```python
from build123d import *

# Parameters (mm, degrees)
SKETCH1_W           = 20.3
SKETCH1_H           = 20.3
BOSS_EXTRUDE1_DEPTH = 39.3
FILLET1_R           = 1
SKETCH2_R           = 1
CUT_EXTRUDE1_DEPTH  = 2.5
SKETCH3_R           = 8
BOSS_EXTRUDE2_DEPTH = 1.5
SKETCH5_R           = 2
BOSS_EXTRUDE3_DEPTH = 20
CUT_EXTRUDE2_START  = -15
CUT_EXTRUDE2_DEPTH  = 15


with BuildPart() as part:
    # Sketch1 → Boss-Extrude1 (new body)
    with BuildSketch(Plane.XY):
        Rectangle(SKETCH1_W, SKETCH1_H)
    extrude(amount=BOSS_EXTRUDE1_DEPTH)

    # Fillet1
    fillet1_edges = [part.edges().sort_by_distance(p)[0] for p in [
        (-10.15, 10.15, 19.65),
        (10.15, 10.15, 19.65),
        (10.15, -10.15, 19.65),
        (-10.15, -10.15, 19.65),
    ]]
    fillet(fillet1_edges, radius=FILLET1_R)

    # Sketch2 → Cut-Extrude1 (cut)
    with BuildSketch(Plane.XY.offset(39.3)):
        with Locations((-7.7, 7.7)):
            Circle(SKETCH2_R)
        with Locations((-7.7, -7.7)):
            Circle(SKETCH2_R)
        with Locations((7.7, -7.7)):
            Circle(SKETCH2_R)
        with Locations((7.7, 7.7)):
            Circle(SKETCH2_R)
    extrude(amount=-CUT_EXTRUDE1_DEPTH, mode=Mode.SUBTRACT)

    # Sketch3 → Boss-Extrude2 (add)
    with BuildSketch(Plane.XY.offset(39.3)):
        Circle(SKETCH3_R)
    extrude(amount=BOSS_EXTRUDE2_DEPTH)

    # Sketch5 → Boss-Extrude3 (add)
    with BuildSketch(Plane.XY.offset(39.3)):
        Circle(SKETCH5_R)
    extrude(amount=BOSS_EXTRUDE3_DEPTH)

    # Sketch6 → Cut-Extrude2 (cut)
    with BuildSketch(Plane.XY.offset(59.3).offset(CUT_EXTRUDE2_START)):
        with BuildLine():
            Line((-1.322875656, 1.5), (1.322875656, 1.5))
            ThreePointArc((1.322875656, 1.5), (0, 2), (-1.322875656, 1.5))
        make_face()
    extrude(amount=CUT_EXTRUDE2_DEPTH, mode=Mode.SUBTRACT)


solid = part.part
```
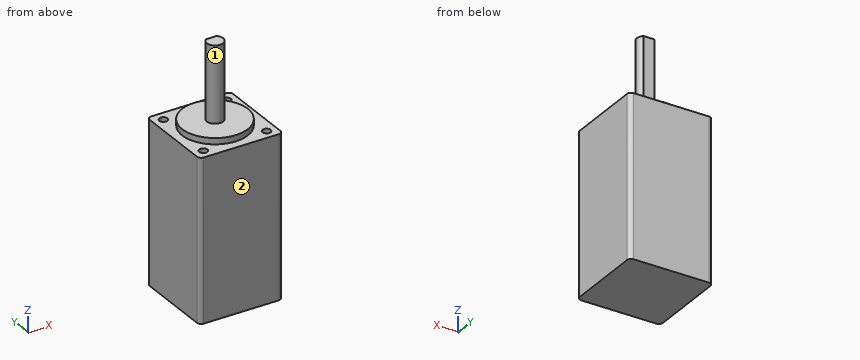
Build history of the part. All positions in model axes, mm. Face numbers are marked on the shaded views. A direction names the side the tool comes from. Give positions to 0.01 mm unless a question says otherwise; leave off trailing zeros. Loops run counter-clockwise (first coordinate to the right, second up) from the corner with the lowest first, then second, coordinate; pieces in that order, holes last. Notation, with made-up numbers: (68.5, 74) - (97.5, 74) arc R11 cw to (97.5, 90) - close; hole circle Ø11 at (53, -19.75). An arc over 180 degrees is marked (long way). Use a Markdown table: item, result.
(1) Drop flat-ended pins along their axis: pin 1 Ø1.6 at (x, y) = (8, -7.5) entering from +Z; pin 2 Ø10 at (x, y) = (4.5, -3) entering from -Z; pin 3 Ø0.6 at (x, y) = (-8, 7.5) entering from +Z; pin 4 Ø1 at (x, y) = (-6.5, 1) entering from +Z. Give the stop position or say it passes through.
Taken from the geometry:
| item | result |
|---|---|
| pin 1 | z = 39.3 |
| pin 2 | z = 0 |
| pin 3 | z = 36.8 |
| pin 4 | z = 40.8 |
(2) Band-saw the part on D-D (x = 3.5). Give the cut face in (y, z).
Taken from the geometry:
| item | result |
|---|---|
| outline | (-10.15, 0) - (10.15, 0) - (10.15, 39.3) - (7.19, 39.3) - (7.19, 40.8) - (-7.19, 40.8) - (-7.19, 39.3) - (-10.15, 39.3) - close |
(3) Band-saw the part on A-A (x = 0). Give the cut face in (y, z), and give its area (3 significant figures).
Taken from the geometry:
| item | result |
|---|---|
| outline | (-10.15, 0) - (10.15, 0) - (10.15, 39.3) - (8, 39.3) - (8, 40.8) - (2, 40.8) - (2, 44.3) - (1.5, 44.3) - (1.5, 59.3) - (-2, 59.3) - (-2, 40.8) - (-8, 40.8) - (-8, 39.3) - (-10.15, 39.3) - close |
| area | 888 mm2 |
(4) Band-saw the part on C-C (z = 54.5). Give the cut face in (x, y).
Taken from the geometry:
| item | result |
|---|---|
| outline | (-1.32, 1.5) arc R2 ccw (long way) to (1.32, 1.5) - close |
(5) Band-saw the part on B-B (y = 0). Give the cut face in (x, z), and give its area (3 significant figures).
Taken from the geometry:
| item | result |
|---|---|
| outline | (-10.15, 0) - (10.15, 0) - (10.15, 39.3) - (8, 39.3) - (8, 40.8) - (2, 40.8) - (2, 59.3) - (-2, 59.3) - (-2, 40.8) - (-8, 40.8) - (-8, 39.3) - (-10.15, 39.3) - close |
| area | 896 mm2 |
(6) Which spindle directions (+Z, -Z, +X, -X, +Y, -Y) get a long thin tool onto all of the face, cutting with end or side? Do the marked faces 1 and 2. Say none if no direction does.
Taken from the geometry:
| item | result |
|---|---|
| face 1 | +Z |
| face 2 | +Z, -Z, +X, -X, -Y |
(7) Wall check: line 1 along Y through (x, z) = (7.7, 38.45); line 2 along Z through (x, y) = (2, -6.75); line 3 along Z through (x, y) = (9.25, -8.5). Give the ranges that are in metal, low to high.
Taken from the geometry:
| item | result |
|---|---|
| line 1 | -10.15 to -8.7, -6.7 to 6.7, 8.7 to 10.15 |
| line 2 | 0 to 40.8 |
| line 3 | 0 to 39.3 |
